Check sheet for the modelled part. Datum: model origin and axes. Units: mm. A direction names the side the tool comes from. Coordinates: 2 decimals unless noted, no trailing zeros. Loops run counter-clockwise (first coordinate to the right, second up) from the corner with the lowest first, then second, coordinate; pieces in that order, holes last.
```python
from build123d import *

# Parameters (mm, degrees)
BOX003_W     = 71
BOX003_H     = 25
BOX003_DEPTH = 50
BOX004_W     = 71
BOX004_H     = 25
BOX004_DEPTH = 50
BOX002_W     = 100
BOX002_H     = 105
BOX002_DEPTH = 30
BOX001_W     = 520
BOX001_H     = 275
BOX001_DEPTH = 140
BOX005_W     = 530
BOX005_H     = 285
BOX005_DEPTH = 144


with BuildPart() as wheelhole1:
    # Box003 → Box003 (new body)
    with BuildSketch(Plane(origin=(450, -1, -1), x_dir=(1, 0, 0), z_dir=(0, 0, 1))):
        with Locations((35.5, 12.5)):
            Rectangle(BOX003_W, BOX003_H)
    extrude(amount=BOX003_DEPTH)


with BuildPart() as wheelhole2:
    # Box004 → Box004 (new body)
    with BuildSketch(Plane(origin=(450, 251, -1), x_dir=(1, 0, 0), z_dir=(0, 0, 1))):
        with Locations((35.5, 12.5)):
            Rectangle(BOX004_W, BOX004_H)
    extrude(amount=BOX004_DEPTH)


with BuildPart() as fusion:
    # Box002 → Box002 (new body)
    with BuildSketch(Plane(origin=(-1, 90, -1), x_dir=(1, 0, 0), z_dir=(0, 0, 1))):
        with Locations((50, 52.5)):
            Rectangle(BOX002_W, BOX002_H)
    extrude(amount=BOX002_DEPTH)

    # Fusion: union wheelhole1, wheelhole2
    add(wheelhole1.part)
    add(wheelhole2.part)


with BuildPart() as cavity:
    # Box001 → Box001 (new body)
    with BuildSketch(Plane.XY):
        with Locations((260, 137.5)):
            Rectangle(BOX001_W, BOX001_H)
    extrude(amount=BOX001_DEPTH)

    # Cut: cut Fusion
    add(fusion.part, mode=Mode.SUBTRACT)


with BuildPart() as suitcase:
    # Box005 → Box005 (new body)
    with BuildSketch(Plane(origin=(-5, -5, -5), x_dir=(1, 0, 0), z_dir=(0, 0, 1))):
        with Locations((265, 142.5)):
            Rectangle(BOX005_W, BOX005_H)
    extrude(amount=BOX005_DEPTH)

    # Cut001: cut cavity
    add(cavity.part, mode=Mode.SUBTRACT)


with BuildPart() as suitcase_1:
    # Cut001 placement: moved
    add(suitcase.part.moved(Location((0, -142.5, 0))))


solid = suitcase_1.part
```
1) Scan lines: line 1 (Y direction, x = 66.5, z = 25); line 2 (X direction, y = 21.5, z = 51.5); line 3 (Y direction, x = 390, z = 102). Record each from-to range of solid material in increasing order.
Answer sheet:
line 1: y = -147.5 to -142.5, -52.5 to 52.5, 132.5 to 137.5
line 2: x = -5 to 0, 520 to 525
line 3: y = -147.5 to -142.5, 132.5 to 137.5
2) Section check D-D on z = 107. Enter the section's corners in (x, y).
Answer sheet:
outline: (-5, -147.5) - (525, -147.5) - (525, 137.5) - (-5, 137.5) - close; hole (0, -142.5) - (520, -142.5) - (520, 132.5) - (0, 132.5) - close
3) Mould release check, pull along X, two halves, no side actions. Record for faces 3 (the flat face through (525, -7, 66)), 4 (the flat face through (485, 121, 49)), 5 (the flat face through (450, -131, 24)), 6 (the flat face through (256, -3, -5)): +X half, -X half, draft (parallel to the pull), parting line (faces both ways), or undercut.
Answer sheet:
face 3: +X half
face 4: undercut
face 5: undercut
face 6: draft
4) Section check A-A on z = 8. Enter the section's corners in (x, y).
Answer sheet:
outline: (-5, -147.5) - (525, -147.5) - (525, 137.5) - (-5, 137.5) - close; hole (0, -142.5) - (450, -142.5) - (450, -118.5) - (520, -118.5) - (520, 108.5) - (450, 108.5) - (450, 132.5) - (0, 132.5) - (0, 52.5) - (99, 52.5) - (99, -52.5) - (0, -52.5) - close
5) Set-up check for faces 1 (the flat face through (485, -118.5, 24)), 2 (the flat face through (256, -147.5, 66)): record each of +Z, -Z, +X, -X, +Y, -Y from which the full face is reachable in a straight line by a thin tool's end or side.
Answer sheet:
face 1: +Z
face 2: +Z, -Z, +X, -X, -Y
6) Depth check by flat-ended pin: pin 1 (2 mm diameter, centred on x = 247, y = -80.5, fed in from +Z); pin 2 (7 mm diameter, centred on x = 476, y = 116, fed in from +Z). Enter the tip coordinate at first touch or a pass-through.
Answer sheet:
pin 1: stops at z = 0
pin 2: stops at z = 49
7) Section check C-C on x = 473. Enter the section's corners in (y, z), plus the area to 3 significant figures.
Answer sheet:
outline: (-147.5, -5) - (137.5, -5) - (137.5, 139) - (132.5, 139) - (132.5, 49) - (108.5, 49) - (108.5, 0) - (-118.5, 0) - (-118.5, 49) - (-142.5, 49) - (-142.5, 139) - (-147.5, 139) - close
area: 5,170 mm2
8) Section check B-B on y = -97.5. Enter the section's corners in (x, z).
Answer sheet:
outline: (-5, -5) - (525, -5) - (525, 139) - (520, 139) - (520, 0) - (0, 0) - (0, 139) - (-5, 139) - close
